Job drawing, mm, ordinate dimensions from the low corner. One solid piece. A direction names the side the tool comes from. Round coordinates to 2 decimals unless told otherwise and drop trailing zeros. Loops run counter-clockwise (first coordinate to the right, second up) from the corner with the lowest first, then second, coordinate; pieces in that order, holes last. Notation, with made-up numbers: M 56.5,89 L 77.5,89 A13 ccw 77.5,103 Z; hole C -19.5,21.25 d8. An arc over 180 degrees is marked long. Put each result on its own line as item: value. Start each with the question number.
1) Slice it at A-A on x = 5. Give the cut face in (y, z), then the cut area to 3 significant figures.
2) Which spindle directions (+Z, -Z, +X, -X, +Y, -Y) get a long thin tool onto all of the face, cutting with end or side? Do the marked faces 1 and 2. Say none if no direction does.
3) Probe line 1 along Z through (x, y) = (5, 2.05); line 2 along Y through (x, z) = (22.7, 5); line 3 along Z through (x, y) = (4.5, 2). List the from-to ranges inside material, lowest first.
4) Drop flat-ended pins along their axis: pin 1 Ø6 at (x, z) = (14.5, 20) entering from +Y; pin 2 Ø1.8 at (y, z) = (12, 5) entering from +X. Give the stop position or say it passes through.
5) Slice it at D-D on z = 27.5. Give the cut face in (x, y), then the cut area to 3 significant figures.
6) Slice it at C-C on x = 21.5. Give the cut face in (y, z), then the cut area to 3 significant figures.
7) Slice it at B-B on z = 5. Give the cut face in (x, y), then the cut area to 3 significant figures.
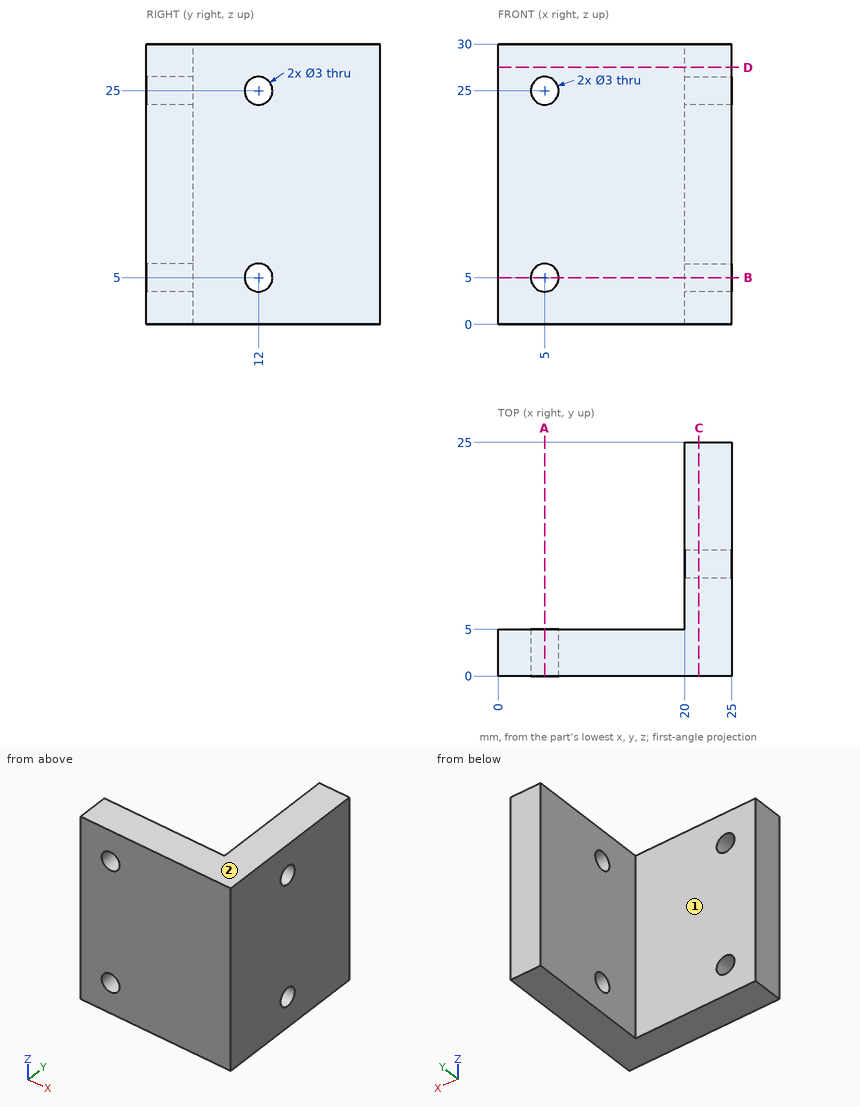
Recorded:
1. outline: M 0,0 L 5,0 L 5,3.5 L 0,3.5 Z; M 0,6.5 L 5,6.5 L 5,23.5 L 0,23.5 Z; M 0,26.5 L 5,26.5 L 5,30 L 0,30 Z
1. area: 120 mm2
2. face 1: +Z, -Z, -X, +Y
2. face 2: +Z, +X, -X, +Y, -Y
3. line 1: z = 0 to 3.5, 6.5 to 23.5, 26.5 to 30
3. line 2: y = 0 to 10.5, 13.5 to 25
3. line 3: z = 0 to 3.59, 6.41 to 23.59, 26.41 to 30
4. pin 1: stops at y = 5
4. pin 2: passes through
5. outline: M 0,0 L 25,0 L 25,25 L 20,25 L 20,5 L 0,5 Z
5. area: 225 mm2
6. outline: M 0,0 L 25,0 L 25,30 L 0,30 Z; hole C 12,5 d3; hole C 12,25 d3
6. area: 736 mm2
7. outline: M 0,0 L 3.5,0 L 3.5,5 L 0,5 Z; M 6.5,0 L 25,0 L 25,10.5 L 20,10.5 L 20,5 L 6.5,5 Z; M 20,13.5 L 25,13.5 L 25,25 L 20,25 Z
7. area: 195 mm2
